Verification items for the finished model (mm, model axes). A direction names the side the tool comes from. Round coordinates to 2 decimals unless told otherwise and drop trailing zeros. Order: outer loops, then holes, each group sorted by start corner. A loop starts at its lowest first (then second) coordinate and runs counter-clockwise, first axis right, second up.
```python
from build123d import *

# Parameters (mm, degrees)
EXTRUDE_1_DEPTH     = 20
CHAMFER_1_SIZE      = 10
CUT_EXTRUDE_2_REACH = 38.056
SKETCH_4_W          = 2.3
SKETCH_4_H          = 5.3
CUT_EXTRUDE_3_DEPTH = 11


with BuildPart() as part:
    # 草圖1 → 填料-伸長1 (new body)
    with BuildSketch(Plane(origin=(0, 0, 0), x_dir=(1, 0, 0), z_dir=(0, 1, 0))):
        with BuildLine():
            Line((0, -4), (0, -21.213203436))
            Line((0, -21.213203436), (-4, -21.213203436))
            Line((-4, -21.213203436), (-21.213203436, -4))
            Line((-21.213203436, -4), (-21.213203436, 0))
            Line((-21.213203436, 0), (-4, 0))
            Line((-4, 0), (-3, 0))
            Line((-3, 0), (-3, -0.267949192))
            ThreePointArc((-3, -0.267949192), (-3.414213562, -3.414213562), (-0.267949192, -3))
            Line((-0.267949192, -3), (0, -3))
            Line((0, -3), (0, -4))
        make_face()
    extrude(amount=EXTRUDE_1_DEPTH)

    # 導角1
    chamfer_1_edges = [part.edges().sort_by_distance(p)[0] for p in [
        (-12.606601718, 0, 12.606601718),
    ]]
    chamfer(chamfer_1_edges, length=CHAMFER_1_SIZE)

    # 草圖3 → 除料-伸長2 (cut, up to next)
    with BuildSketch(Plane.ZY.offset(21.213203436), mode=Mode.PRIVATE) as cut_extrude_2_sk1:
        with BuildLine():
            Line((3, 19.732050808), (3, 20))
            Line((3, 20), (0, 20))
            Line((0, 20), (0, 17))
            Line((0, 17), (0.267949192, 17))
            ThreePointArc((0.267949192, 17), (3.414213562, 16.585786438), (3, 19.732050808))
        make_face()
    cut_extrude_2_tool1 = extrude(cut_extrude_2_sk1.sketch, amount=-CUT_EXTRUDE_2_REACH, mode=Mode.PRIVATE) & part.part
    cut_extrude_2 = cut_extrude_2_tool1.solids().sort_by_distance((-21.213203, 18.105499, 1.894501))[0]
    add(cut_extrude_2, mode=Mode.SUBTRACT)

    # 鏡射1: 除料-伸長2 across plane
    add(cut_extrude_2.mirror(Plane(origin=(0, 0, 0), x_dir=(-0.7071067811865478, 0, 0.7071067811865472), z_dir=(0.7071067811865475, 0, 0.7071067811865477))), mode=Mode.SUBTRACT)

    # 草圖4 → 除料-伸長3 (cut)
    with BuildSketch(Plane.XZ):
        with Locations((-2.15, 7.563203436)):
            Rectangle(SKETCH_4_W, SKETCH_4_H)
    cut_extrude_3 = extrude(amount=-CUT_EXTRUDE_3_DEPTH, mode=Mode.SUBTRACT)

    # 鏡射2: 除料-伸長3 across plane
    add(cut_extrude_3.mirror(Plane(origin=(0, 0, 0), x_dir=(-0.7071067811865478, 0, 0.7071067811865472), z_dir=(0.7071067811865475, 0, 0.7071067811865477))), mode=Mode.SUBTRACT)

    # 草圖5 → 除料-旋轉1 (revolve, cut)
    with BuildSketch(Plane(origin=(0, 18, 0), x_dir=(1, 0, 0), z_dir=(0, 1, 0))):
        with BuildLine():
            Line((10, 0), (-10, 0))
            ThreePointArc((-10, 0), (0, -10), (10, 0))
        make_face()
    revolve(axis=Axis((10, 18, 0), (-1, 0, 0)), mode=Mode.SUBTRACT)


solid = part.part
```
1) Sectioned sample at A-A on z = 5.5. Record the cut outline in (x, y).
2) Go/stop test with flat-tipped pins: pin 1 Ø3 at (x, z) = (-18.5, 6) entering from -Y; pin 2 Ø0.7 at (y, z) = (6, 2.5) entering from -X; pin 3 Ø2 at (x, y) = (-5, 18) entering from -Z; pin 4 Ø3 at (x, y) = (-2, 18) entering from +Z. Record where each tip stops, or that it passes through.
3) Draft check along X on faces 1 (the flat face through (-2, 11, 8)), 2 (the flat face through (0, 8, 12)), 3 (the flat face through (-3.7, 19.4, 21.213)). Enter one of: released by +X, released by -X, zero draft, split by the parting line, or undercut.
4) Sectioned sample at C-C on x = -2. Record the cut outline in (y, z).
5) Sectioned sample at D-D on y = 5.25. Record the cut outline in (x, z).
6) Tool access check on faces 4 (the flat face through (-2, 5, 4.913)), 5 (the flat face through (-1, 5, 8)), 6 (the flat face through (-8, 11, 2)). Record the directions out of +Z, -Z, +X, -X, +Y, -Y that give a thin tool (end or side, any length) a straight path to the whole face; none if there is none.
7) Scan lines: probe 1 along Z at (x, y) = (-2, 5.25); probe 2 along Z at (x, y) = (-7.5, 10.25); probe 3 along X at (y, z) = (2.75, 2). Record each from-to range of solid material in increasing order.
8) Sectioned sample at B-B on y = 16.5. Record the cut outline in (x, z), then the cut area to 3 significant figures.
Returned:
1. outline: (-19.71, 10) - (-5.57, 0) - (-3.3, 0) - (-3.3, 10.33) arc R8.35 cw to (-8.11, 20) - (-19.71, 20) - close; (-1, 0) - (0, 0) - (0, 9.65) arc R8.35 cw to (-1, 9.71) - close
2. pin 1: stops at y = 8
2. pin 2: stops at x = -17.66
2. pin 3: stops at z = 8
2. pin 4: passes through
3. face 1: undercut
3. face 2: released by +X
3. face 3: zero draft
4. outline: (0, 4) - (9.06, 4) arc R9.8 cw to (9.52, 4.91) - (0, 4.91) - close; (0.81, 10.21) - (11, 10.21) - (11, 6.86) arc R9.8 cw to (16, 9.59) - (16, 21.21) - (8.59, 21.21) - close
5. outline: (-18.5, 0) - (-3, 0) - (-3, 0.27) arc R2 cw (long way) to (-0.27, 3) - (0, 3) - (0, 18.5) - close; hole (-10.21, 1) - (-4.91, 1) - (-4.91, 3.3) - (-10.21, 3.3) - close; hole (-3.3, 4.91) - (-1, 4.91) - (-1, 10.21) - (-3.3, 10.21) - close
6. face 4: +Y, -Y
6. face 5: -Y
6. face 6: +X, -Y
7. probe 1: z = 4 to 4.91, 10.21 to 16.5
7. probe 2: z = 0 to 1, 3.3 to 17.71
7. probe 3: x = -12.96 to -10.21, -4.91 to -4
8. outline: (-21.21, 0) - (-9.89, 0) arc R9.89 cw to (-9.86, 0.68) - (-21.21, 0.68) - close; (-21.21, 3.32) - (-9.31, 3.32) arc R9.89 cw to (-3.32, 9.31) - (-3.32, 21.21) - (-4, 21.21) - (-21.21, 4) - close; (-0.68, 9.86) arc R9.89 cw to (0, 9.89) - (0, 21.21) - (-0.68, 21.21) - close
8. area: 164 mm2
